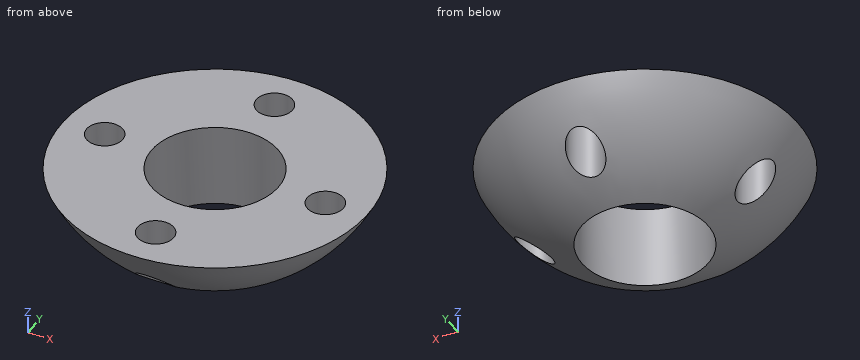
from build123d import *

# Parameters (mm, degrees)
F3_DEPTH = 18
F4_R     = 1.905
F4_R_2   = 6.6675
F5_DEPTH = 10.001


# Not quite as in the source:
# - a feature names something its author has since deleted; it is built from what else it names


with BuildPart() as f1:
    # F0 (on Front) → F1 (revolve)
    with BuildSketch(Plane.XZ):
        with BuildLine():
            Line((0, 18), (0, -18))
            ThreePointArc((0, -18), (18, 0), (0, 18))
        make_face()
    revolve(axis=Axis((0, 0, 0), (0, 0, -1)))

    # F2 (on Right) → F3 (cut, symmetric)
    with BuildSketch(Plane.YZ):
        with BuildLine():
            Line((-16.1245154966, -8), (16.1245154966, -8))
            ThreePointArc((16.1245154966, -8), (0, 18), (-16.1245154966, -8))
        make_face()
    extrude(amount=F3_DEPTH, both=True, mode=Mode.SUBTRACT)

    # F4 (on face) → F5 (cut, through all)
    with BuildSketch(Plane.XY.offset(-8)):
        with Locations((0, -11.7475)):
            Circle(F4_R)
        with Locations((11.7475, 0)):
            Circle(F4_R)
        with Locations((0, 11.7475)):
            Circle(F4_R)
        with Locations((-11.7475, 0)):
            Circle(F4_R)
        Circle(F4_R_2)
    extrude(amount=-F5_DEPTH, mode=Mode.SUBTRACT)


solid = f1.part
Source: CAD feature listing. Evaluate the final solid. Frame: model axes, mm. Round coordinates to 2 decimals unless told otherwise and drop trailing zeros. Loops run counter-clockwise (first coordinate to the right, second up) from the corner with the lowest first, then second, coordinate; pieces in that order, holes last. Notation, with made-up numbers: (53.5, 64.25) -> (93.5, 64.25) arc R27 cw to (93.5, 100.25) -> close; hole circle Ø5 at (-8, 7.5). An arc over 180 degrees is marked (long way). Answer as a JSON object with one key per item and string values. Group by question number.
Q1. Section query A-A (y = 0). Output: boundary loops of the cut face in (x, z).
Q2. Section query D-D (y = 12.5). Output: boundary loops of the cut face in (x, z).
Q3. Contact query for flat-ended pins moving along their axis: P1, Ø8, axis at x = 0, y = 0, coming from the +Z side; P2, Ø2, axis at y = -0.5, z = -13.5, coming from the +X side; P3, Ø5, axis at x = 0, y = -11.75, coming from the -Z side; P4, Ø6, axis at x = -11.75, y = 0, coming from the +Z side. Output: stop coordinate, or through.
Q4. Section query C-C (z = -11). Output: boundary loops of the cut face in (x, y) (1 decimal), plus the area to 3 significant figures.
Q5. Ray query, line 1 (X direction, y = -0.5, z = -10.5); line 2 (Y direction, x = 0, z = -10.5); line 3 (Y direction, x = 0, z = -9.75). Return the intervals inside material, ascending. Write a range as from..to.
Completed:
{
 "1": {"outline": "(-16.12, -8) arc R18 ccw to (-13.65, -11.73) -> (-13.65, -8) -> close; (-9.84, -15.07) arc R18 ccw to (-6.67, -16.72) -> (-6.67, -8) -> (-9.84, -8) -> close; (6.67, -16.72) arc R18 ccw to (9.84, -15.07) -> (9.84, -8) -> (6.67, -8) -> close; (13.65, -11.73) arc R18 ccw to (16.12, -8) -> (13.65, -8) -> close"},
 "2": {"outline": "(-10.19, -8) arc R12.95 ccw to (-1.75, -12.83) -> (-1.75, -8) -> close; (1.75, -12.83) arc R12.95 ccw to (10.19, -8) -> (1.75, -8) -> close"},
 "3": {"P1": "through", "P2": "x = 10.57", "P3": "z = -15.44", "P4": "z = -8"},
 "4": {"outline": "circle Ø28.5 at (0, 0); hole circle Ø3.8 at (-11.7, 0); hole circle Ø13.3 at (0, 0); hole circle Ø3.8 at (0, -11.7); hole circle Ø3.8 at (0, 11.7); hole circle Ø3.8 at (11.7, 0)", "area": "452 mm²"},
 "5": {"line 1": "-14.61..-13.59, -9.91..-6.65, 6.65..9.91, 13.59..14.61", "line 2": "-14.62..-13.65, -9.84..-6.67, 6.67..9.84, 13.65..14.62", "line 3": "-15.13..-13.65, -9.84..-6.67, 6.67..9.84, 13.65..15.13"}
}
